```python
from build123d import *

# Parameters (mm, degrees)
F0_R            = 76.2
F1_DEPTH        = 12.7
F2_R            = 16.51
F3_DEPTH        = 4.7625
F3_COPIES_COUNT = 5
F4_R            = 16.51
F5_DEPTH        = 4.7625


# Not quite as in the source:
# - a pattern or mirror of a feature is missing from the dataset's text; its kind, count and spacing are read off the source's solid


with BuildPart() as f1:
    # F0 (on Top) → F1 (new body)
    with BuildSketch(Plane.XY):
        Circle(F0_R)
    extrude(amount=F1_DEPTH)

    # F2 (on face) → F3 (cut)
    with BuildSketch(Plane.XY.offset(12.7)):
        with Locations((0, 45.9601860202)):
            Circle(F2_R)
    f3 = extrude(amount=-F3_DEPTH, mode=Mode.SUBTRACT)

    # F3_copies: F3 ×5 about axis
    f3_copies_axis = Axis((0, 0, 0), (0, 0, 1))
    for i in range(1, F3_COPIES_COUNT):
        add(f3.rotate(f3_copies_axis, i * 360 / F3_COPIES_COUNT), mode=Mode.SUBTRACT)

    # F4 (on face) → F5 (cut)
    with BuildSketch(Plane.XY.offset(12.7)):
        Circle(F4_R)
    extrude(amount=-F5_DEPTH, mode=Mode.SUBTRACT)


solid = f1.part
```
Part model, mm, in its own coordinate system. A direction names the side the tool comes from. Round coordinates to 2 decimals unless told otherwise and drop trailing zeros. Order: outer loops, then holes, each group sorted by start corner. A loop starts at its lowest first (then second) coordinate and runs counter-clockwise, first axis right, second up. Notation, with made-up numbers: M 62.25,-22.5 L 108.25,-22.5 A8 ccw 108.25,-14.5 Z; hole C -32.75,-14 d10. An arc over 180 degrees is marked long. Put each result on its own line as item: value. Start each with the question number.
1. Two-plate mould, pull along Y, no slides. Class faces 3 (the face through (30.11, 23.56, 10.35)), 4 (the face through (-60.47, -46.367, 6.261)), 5 (the face through (-1, 18, 12.7)): +Y half, -Y half, draft (parallel to the pull), parting line (faces both ways), or undercut.
2. Drop flat-ended pins along their axis: pin 1 (10 mm diameter, centred on x = -3, y = 1, fed in from +Z); pin 2 (6 mm diameter, centred on y = 59, z = 9.5, fed in from -X); pin 3 (3 mm diameter, centred on y = -51.5, z = 11, fed in from -X). Give the stop position or say it passes through.
3. Drill centre lines: probe 1 along X at (y, z) = (1.5, 10.5); probe 2 along X at (y, z) = (-44.5, 9.5); probe 3 along Z at (x, y) = (5, 8). Where is each one in solid material? Low to high. Write a range as [from, to].
4. Tool access for faces 1 (the face through (-1, 1, 0)), 2 (the face through (44, 14, 7.937)): list every direction of +Z, -Z, +X, -X, +Y, -Y with a clear straight run to the whole face (end or side of a thin tool).
5. Slice it at C-C on z = 10.25. List the corners of the cut face in (x, y), then the cut area to 3 significant figures.
6. Slice it at A-A on x = 0. List the corners of the cut face in (y, z).
7. Slice it at D-D on x = -31. List the corners of the cut face in (y, z).
8. Slice it at B-B on y = 9. List the corners of the cut face in (x, z), then the cut area to 3 significant figures.
Findings:
1. face 3: undercut
1. face 4: parting line
1. face 5: draft
2. pin 1: z = 7.94
2. pin 2: x = -51.68
2. pin 3: x = -57.5
3. probe 1: [-76.19, -54.26], [-33.16, -16.44], [16.44, 33.16], [54.26, 76.19]
3. probe 2: [-61.86, -41.81], [-12.21, 12.21], [41.81, 61.86]
3. probe 3: [0, 7.94]
4. face 1: -Z, +X, -X, +Y, -Y
4. face 2: +Z
5. outline: C 0,0 d152.4; hole C -43.71,14.2 d33.02; hole C -27.01,-37.18 d33.02; hole C 0,0 d33.02; hole C 0,45.96 d33.02; hole C 27.01,-37.18 d33.02; hole C 43.71,14.2 d33.02
5. area: 13,100 mm2
6. outline: M -76.2,0 L 76.2,0 L 76.2,12.7 L 62.47,12.7 L 62.47,7.94 L 29.45,7.94 L 29.45,12.7 L 16.51,12.7 L 16.51,7.94 L -16.51,7.94 L -16.51,12.7 L -76.2,12.7 Z
7. outline: M -69.61,0 L 69.61,0 L 69.61,12.7 L 24.74,12.7 L 24.74,7.94 L 3.67,7.94 L 3.67,12.7 L -21.16,12.7 L -21.16,7.94 L -53.2,7.94 L -53.2,12.7 L -69.61,12.7 Z
8. outline: M -75.67,0 L 75.67,0 L 75.67,12.7 L 59.38,12.7 L 59.38,7.94 L 28.04,7.94 L 28.04,12.7 L 13.84,12.7 L 13.84,7.94 L -13.84,7.94 L -13.84,12.7 L -28.04,12.7 L -28.04,7.94 L -59.38,7.94 L -59.38,12.7 L -75.67,12.7 Z
8. area: 1,490 mm2
